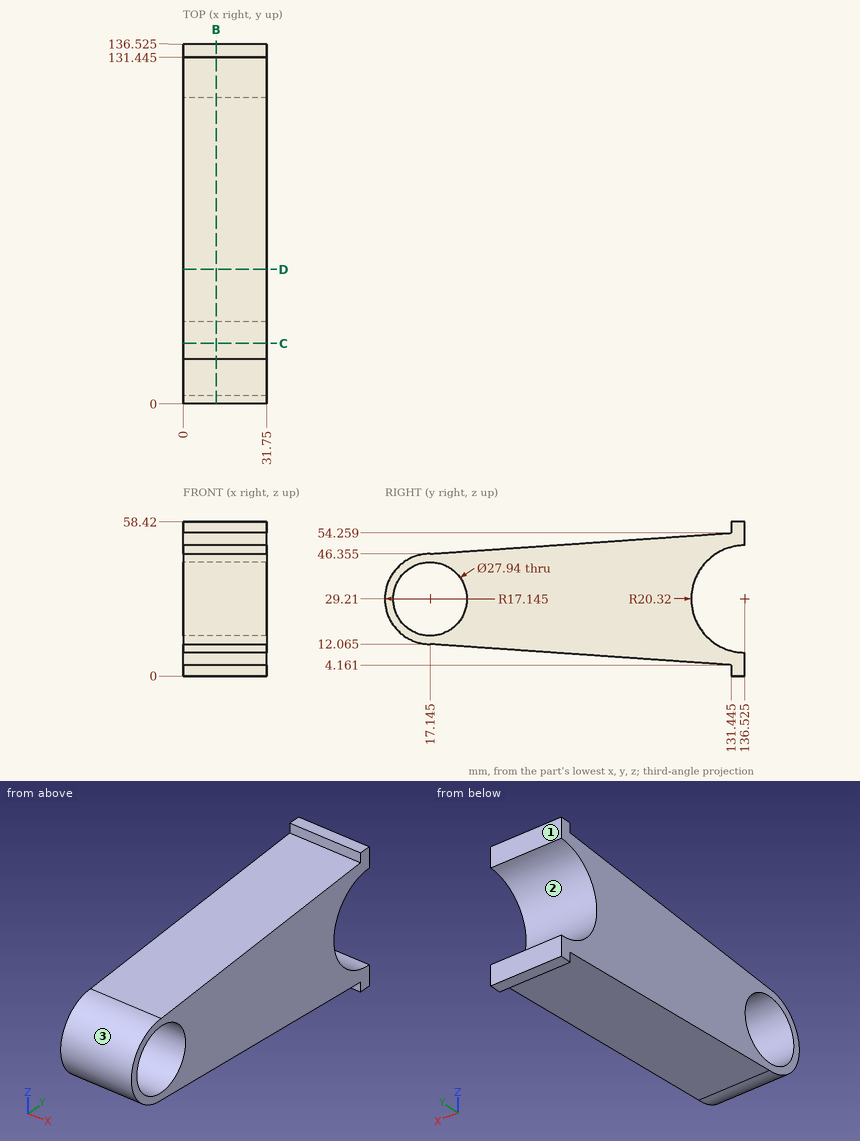
Here's the drawing with two shaded views (mm, measured from the low corner). I have some questions. Give positions to 0.01 mm unless a question says otherwise; leave off trailing zeros. Order: outer loops, then holes, each group sorted by start corner. A loop starts at its lowest first (then second) coordinate and runs counter-clockwise, first axis right, second up.
Q1. Suppose I cut it at D-D, the plane y = 51. Write out the boundary of the cut face in (x, z).
Q2. We'd pull the mould along Z, two halves only. Please class the marked faces 1, 2 and 3: +Z half, -Z half, draft (parallel to the pull), parting line (faces both ways), or undercut.
Q3. Suppose I cut it at B-B, the plane x = 12.5. Write out the boundary of the cut face in (y, z) (1 decimal).
Q4. Suppose I cut it at C-C, the plane y = 23. Write out the boundary of the cut face in (x, z).
Q5. I'm going to push flat-ended pins straight in: P1, Ø1.5, axis at x = 12, y = 67, coming from the +Z side; P2, Ø6, axis at x = 14.5, z = 13, coming from the -Y side (1 decimal); P3, Ø1.2, axis at x = 12, z = 1.5, coming from the -Y side (3 decimals). Where does each tip first touch, or does it pass through?
Q6. If I drill on line 1 along Y through (x, z) = (22, 29.21) (1 decimal); line 2 along Z through (x, y) = (22, 8.5) (1 decimal); line 3 along Y through (x, z) = (12.5, 3) (1 decimal), over which ranges is the centre line in solid material (lowest first)?
Solution:
1. outline: (0, 9.72) - (31.75, 9.72) - (31.75, 48.7) - (0, 48.7) - close
2. face 1: draft
2. face 2: undercut
2. face 3: parting line
3. outline: (17.1, 12.1) - (131.4, 4.2) - (131.4, 0) - (136.5, 0) - (136.5, 8.9) arc R20.3 cw to (136.5, 49.5) - (136.5, 58.4) - (131.4, 58.4) - (131.4, 54.3) - (17.1, 46.4) arc R17.1 ccw to start; hole circle Ø27.9 at (17.1, 29.2)
4. outline: (0, 11.66) - (31.75, 11.66) - (31.75, 16.53) - (0, 16.53) - close; (0, 41.89) - (31.75, 41.89) - (31.75, 46.76) - (0, 46.76) - close
5. P1: stops at z = 49.85
5. P2: stops at y = 6.2
5. P3: stops at y = 131.445
6. line 1: y = 0 to 3.2, 31.1 to 116.2
6. line 2: z = 14.4 to 18.2, 40.2 to 44
6. line 3: y = 131.4 to 136.5
